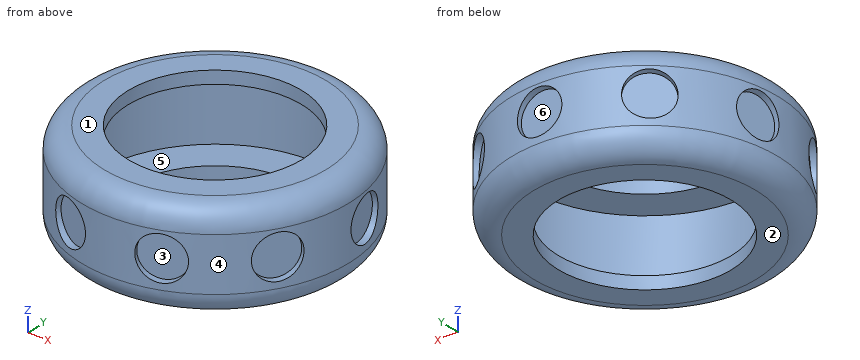
```python
from build123d import *

# Parameters (mm, degrees)
SKETCH5_R           = 30
BOSS_EXTRUDE2_DEPTH = 22
SKETCH6_R           = 19.5
CUT_EXTRUDE3_DEPTH  = 22
SHELL4_T            = -2.84
FILLET2_R           = 5
SKETCH7_R           = 4.938582487
CUT_EXTRUDE4_DEPTH  = 22
CIRPATTERN1_COUNT   = 9


with BuildPart() as part:
    # Sketch5 → Boss-Extrude2 (new body)
    with BuildSketch(Plane.XY):
        Circle(SKETCH5_R)
    extrude(amount=BOSS_EXTRUDE2_DEPTH)

    # Sketch6 → Cut-Extrude3 (cut)
    with BuildSketch(Plane.XY):
        Circle(SKETCH6_R)
    extrude(amount=CUT_EXTRUDE3_DEPTH, mode=Mode.SUBTRACT)

    # Shell4
    shell4_openings = [part.faces().sort_by_distance(p)[0] for p in [
        (-19.5, 0, 11),
    ]]
    offset(amount=SHELL4_T, openings=shell4_openings, kind=Kind.INTERSECTION)

    # Fillet2
    fillet2_edges = [part.edges().sort_by_distance(p)[0] for p in [
        (-30, 0, 0),
        (-30, 0, 22),
    ]]
    fillet(fillet2_edges, radius=FILLET2_R)

    # Sketch7 → Cut-Extrude4 (cut)
    with BuildSketch(Plane(origin=(0, 28.5, 0), x_dir=(1, 0, 0), z_dir=(0, 1, 0))):
        with Locations(Location((0, -11.372504627, 0), (0, 0, 90))):
            Circle(SKETCH7_R)
    cut_extrude4 = extrude(amount=CUT_EXTRUDE4_DEPTH, mode=Mode.SUBTRACT)

    # CirPattern1: Cut-Extrude4 ×9 about axis
    cirpattern1_axis = Axis((0, 0, 0), (0, 0, 1))
    for i in range(1, CIRPATTERN1_COUNT):
        add(cut_extrude4.rotate(cirpattern1_axis, i * 360 / CIRPATTERN1_COUNT), mode=Mode.SUBTRACT)


solid = part.part
```
Geometry check sheet. Reference: the model listing, model coordinates, mm. Face numbers are marked on the shaded views. A direction names the side the tool comes from. Round coordinates to 2 decimals unless told otherwise and drop trailing zeros. Use a Markdown table: item, result. Add a question column.
1) Mould release check, pull along Z, two halves, no side actions. Record for the marked faces 1, 2 and 3: released by +Z, released by -Z, zero draft, split by the parting line, or undercut.
2) Thickness scan on line 1 along Y through (x, z) = (0, 12.25); line 2 along Z through (x, y) = (-5.5, 20); line 3 along Y through (x, z) = (15, 10.5). Record the ranges inside material, lowest first.
3) Gauge pin test, flat ends, axial feed: P1, Ø12, axis at y = -6.5, z = 20, coming from the +X side; P2, Ø5, axis at x = -7.5, z = 18, coming from the -Y side; P3, Ø8, axis at y = -23.5, z = 12.5, coming from the -X side. Record the tip position at first contact, or that the pin passes through.
4) Set-up check for the marked faces 4, 5 and 6: record each of +Z, -Z, +X, -X, +Y, -Y from which the full face is reachable in a straight line by a thin tool's end or side.
Established:
| question | item | result |
|---|---|---|
| 1 | face 1 | released by +Z |
| 1 | face 2 | released by -Z |
| 1 | face 3 | undercut |
| 2 | line 1 | -30 to -27.16, 27.16 to 28.5 |
| 2 | line 2 | 0 to 2.84, 19.16 to 22 |
| 2 | line 3 | -25.98 to -22.64, 22.64 to 24.62, 25.44 to 25.98 |
| 3 | P1 | x = 29.97 |
| 3 | P2 | y = -29.55 |
| 3 | P3 | x = -22.8 |
| 4 | face 4 | +Z, -Z |
| 4 | face 5 | none |
| 4 | face 6 | +Y |
